Geometry: final body of the model. Coordinates: model frame, mm. Round coordinates to 2 decimals unless told otherwise and drop trailing zeros. Loops run counter-clockwise (first coordinate to the right, second up) from the corner with the lowest first, then second, coordinate; pieces in that order, holes last. Notation, with made-up numbers: (18, 52.5) - (33, 52.5) arc R20 ccw to (33, 76.5) - close; hole circle Ø10 at (20, 30.5). An arc over 180 degrees is marked (long way). Answer as a JSON object with one key per item and string values. Group by question number.
Item 1: Section A-A (x = -127). Return the cut outline in (y, z) (1 decimal).
Item 2: First-contact query: pin 1 (13.5 mm diameter, centred on x = -127, y = 25.4, fed in from +Z). Flat tip, straight axial feed; report the tip coordinate or a pass-through.
Item 3: Line query: line 1 (X direction, y = 38, z = 1.5); line 2 (X direction, y = 25.4, z = 23.6); line 3 (Z direction, x = -248.5, y = 13.5) (3 decimals). Output: solid intervals per line, ascending.
Item 4: Section C-C (y = 23.5). Return the cut outline in (x, z) (3 decimals).
Item 5: Section B-B (z = 11.5). Return the cut outline in (x, y) (3 decimals), plus the area to 3 significant figures.
Item 6: Section D-D (x = -354). Return the cut outline in (y, z) (3 decimals).
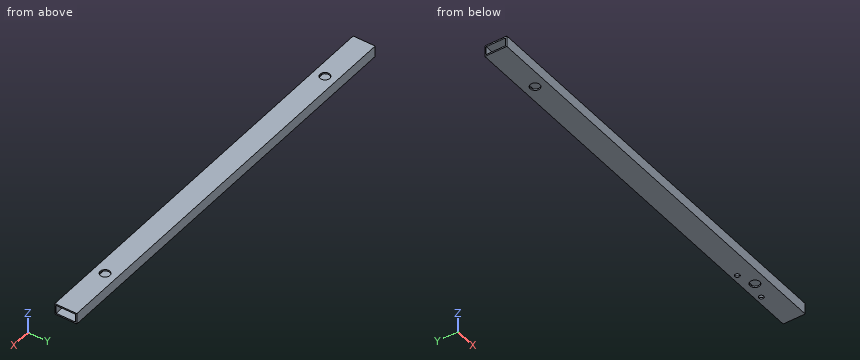
Autodesk Inventor part; units mm, degrees
ref_plane "YZ Plane" through (0, 0, 0) normal (1, 0, 0) x (0, 1, 0)
ref_plane "XZ Plane" through (0, 0, 0) normal (0, 1, 0) x (-1, 0, 0)
ref_plane "XY Plane" through (0, 0, 0) normal (0, 0, 1) x (1, 0, 0)
sketch "Sketch1" plane through (0, 0, 0) normal (0, 0, 1) x (1, 0, 0)
  line L0 (0, 0) -> (-965.2, 0)
  line L1 (-965.2, 0) -> (-965.2, 50.8)
  line L2 (-965.2, 50.8) -> (0, 50.8)
  line L3 (0, 50.8) -> (0, 0)
  dimension "d0" = 50.8
  dimension "d1" = 965.2
extrude "Extrusion1" add sketch "Sketch1" along normal blind 25.4
sketch "Sketch2" plane through (0, 0, 0) normal (1, 0, 0) x (0, 0, -1)
  line L0 (-3.175, 3.175) -> (-22.225, 3.175)
  line L1 (-22.225, 3.175) -> (-22.225, 47.625)
  line L2 (-22.225, 47.625) -> (-3.175, 47.625)
  line L3 (-3.175, 47.625) -> (-3.175, 3.175)
  line L4 (0, 0) -> (-25.4, 0)
  line L5 (0, 50.8) -> (0, 0)
  line L6 (0, 50.8) -> (-25.4, 50.8)
  line L7 (-25.4, 0) -> (-25.4, 50.8)
  dimension "d5" = 3.175
  dimension "d7" = 3.175
  dimension "d8" = 3.175
  dimension "d9" = 3.175
extrude "Extrusion2" cut sketch "Sketch2" against normal blind 965.2 contours L0 L1 L2 L3
sketch "Sketch3" plane through (0, 0, 25.4) normal (0, 0, 1) x (1, 0, 0)
  circle A0 centre (-838.2, 25.4) radius 6.2992
  line L0 (-965.2, 0) -> (0, 0)
  line L1 (-965.2, 0) -> (0, 0)
  line L2 (-965.2, 50.8) -> (-965.2, 0)
  line L3 (0, 0) -> (0, 50.8)
  circle A1 centre (-127, 25.4) radius 11.1125
  dimension "d13" = 25.4
  dimension "d14" = 12.5984
  dimension "d16" = 127
  dimension "d18" = 22.225
hole "Hole1" at (-838.2, 25.4, 25.4) at (-127, 25.4, 25.4) direction (0, 0, -1) diameter 22.225 end through all
sketch "Sketch4" plane through (0, 0, 0) normal (0, 0, -1) x (-1, 0, 0)
  circle A0 centre (165.735, 38.2537) radius 5.5563
  arc A1 (85.416, 33.4832) -> (85.0155, 42.761) centre (88.5446, 38.2658) ccw
  circle A2 centre (165.735, 38.2537) radius 5.5563
  circle A3 centre (88.265, 38.2537) radius 5.5565
  circle A4 centre (88.265, 38.2537) radius 5.5565
  point P0 (0, 0)
extrude "Extrusion3" cut sketch "Sketch4" against normal blind 5.08 contours A0 | A3
Values:
{
 "1": {"outline": "(0, 0) - (14.3, 0) - (14.3, 3.2) - (3.2, 3.2) - (3.2, 22.2) - (14.3, 22.2) - (14.3, 25.4) - (0, 25.4) - close; (36.5, 0) - (50.8, 0) - (50.8, 25.4) - (36.5, 25.4) - (36.5, 22.2) - (47.6, 22.2) - (47.6, 3.2) - (36.5, 3.2) - close"},
 "2": {"pin 1": "passes through"},
 "3": {"line 1": "x = -965.2 to -171.29, -160.18 to -93.82, -82.71 to 0", "line 2": "x = -965.2 to -849.31, -827.09 to -138.11, -115.89 to 0", "line 3": "z = 0 to 3.175, 22.225 to 25.4"},
 "4": {"outline": "(-965.2, 0) - (-849.149, 0) - (-849.149, 3.175) - (-965.2, 3.175) - close; (-965.2, 22.225) - (-849.149, 22.225) - (-849.149, 25.4) - (-965.2, 25.4) - close; (-827.251, 0) - (-137.949, 0) - (-137.949, 3.175) - (-827.251, 3.175) - close; (-827.251, 22.225) - (-137.949, 22.225) - (-137.949, 25.4) - (-827.251, 25.4) - close; (-116.051, 0) - (0, 0) - (0, 3.175) - (-116.051, 3.175) - close; (-116.051, 22.225) - (0, 22.225) - (0, 25.4) - (-116.051, 25.4) - close"},
 "5": {"outline": "(-965.2, 0) - (0, 0) - (0, 3.175) - (-965.2, 3.175) - close; (-965.2, 47.625) - (0, 47.625) - (0, 50.8) - (-965.2, 50.8) - close", "area": "6,130 mm^2"},
 "6": {"outline": "(0, 0) - (50.8, 0) - (50.8, 25.4) - (0, 25.4) - close; hole (3.175, 3.175) - (47.625, 3.175) - (47.625, 22.225) - (3.175, 22.225) - close"}
}
